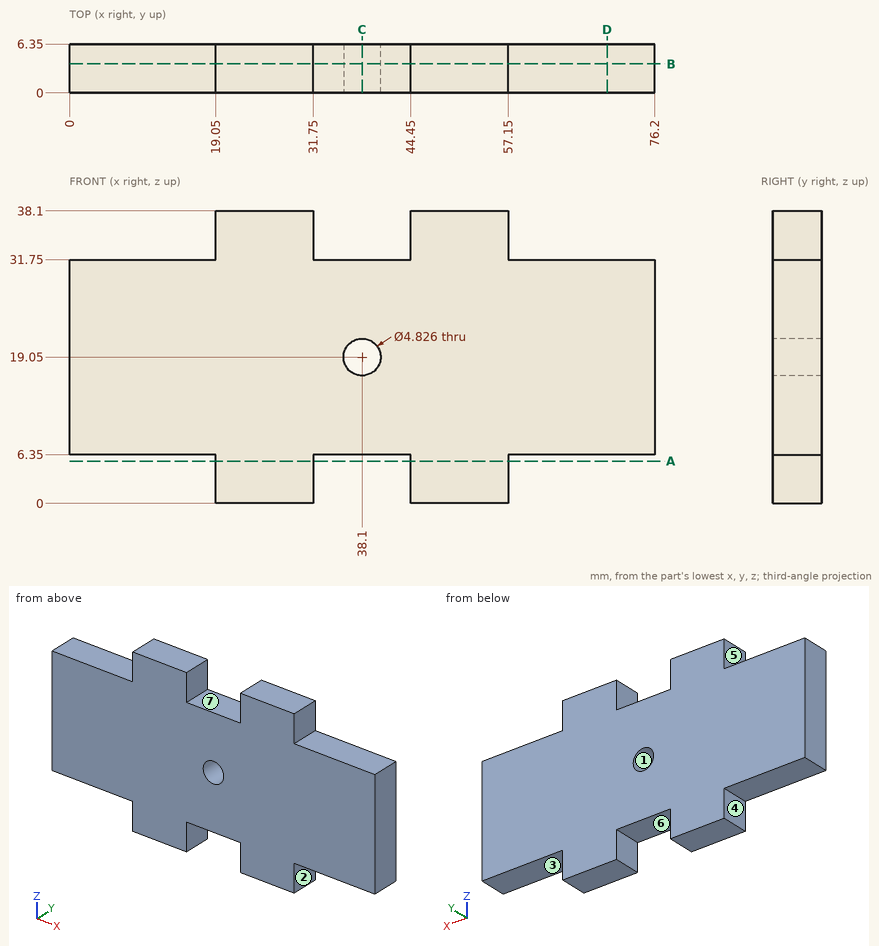
Geometry check sheet. Reference: drawing and pictorial views, mm from the part's lowest x, y, z. A direction names the side the tool comes from. Coordinates: 2 decimals unless noted, no trailing zeros. Write each loop counter-clockwise with the first axis right and the second up, starting at its lowest first coordinate (ties: lowest second). Pieces come first, ordered by that corner, then holes. Notation, with made-up numbers: (-23.75, 4.25) - (33.25, 4.25) arc R7 ccw to (33.25, 17.25) - close; hole circle Ø8 at (-7, 85.5). An arc over 180 degrees is marked (long way). One line per question, with ' | ' between items. Start each with the question number.
1. Draft check along X on the marked faces 1, 2 and 3. Enter one of: released by +X, released by -X, zero draft, split by the parting line, or undercut.
2. Material ranges on line 1 along Z through (x, y) = (38.1, 4); line 2 along X through (y, z) = (5, 4.5); line 3 along X through (y, z) = (4.75, 19.05), recorded low to high.
3. Access from +Z, -Z, +X, -X, +Y, -Y to the whole of each face (thin tool, end or side, straight path). Record for the marked faces 4, 5, 6 and 7.
4. Gauge pin test, flat ends, axial feed: P1, Ø3, axis at x = 70, y = 2, coming from the -Z side; P2, Ø4.5, axis at x = 38.1, z = 19.05, coming from the -Y side; P3, Ø1.9, axis at x = 69, y = 3.5, coming from the +Z side; P4, Ø3, axis at y = 4, z = 2.5, coming from the +X side. Record the tip position at first contact, or that the pin passes through.
5. Section check A-A (z = 5.5). Enter the section's corners in (x, y), plus the area to 3 significant figures.
6. Section check D-D (x = 70). Enter the section's corners in (y, z), plus the area to 3 significant figures.
7. Section check B-B (y = 3.75). Enter the section's corners in (x, z).
8. Section check C-C (x = 38.1). Enter the section's corners in (y, z), plus the area to 3 significant figures.
Computed values:
1) face 1: undercut | face 2: released by +X | face 3: zero draft
2) line 1: 6.35 to 16.64, 21.46 to 31.75 | line 2: 19.05 to 31.75, 44.45 to 57.15 | line 3: 0 to 35.69, 40.51 to 76.2
3) face 4: -Z, -X, +Y, -Y | face 5: +Z, -X, +Y, -Y | face 6: -Z, +Y, -Y | face 7: +Z, +Y, -Y
4) P1: z = 6.35 | P2: through | P3: z = 31.75 | P4: x = 57.15
5) outline: (19.05, 0) - (31.75, 0) - (31.75, 6.35) - (19.05, 6.35) - close; (44.45, 0) - (57.15, 0) - (57.15, 6.35) - (44.45, 6.35) - close | area: 161 mm²
6) outline: (0, 6.35) - (6.35, 6.35) - (6.35, 31.75) - (0, 31.75) - close | area: 161 mm²
7) outline: (0, 6.35) - (19.05, 6.35) - (19.05, 0) - (31.75, 0) - (31.75, 6.35) - (44.45, 6.35) - (44.45, 0) - (57.15, 0) - (57.15, 6.35) - (76.2, 6.35) - (76.2, 31.75) - (57.15, 31.75) - (57.15, 38.1) - (44.45, 38.1) - (44.45, 31.75) - (31.75, 31.75) - (31.75, 38.1) - (19.05, 38.1) - (19.05, 31.75) - (0, 31.75) - close; hole circle Ø4.83 at (38.1, 19.05)
8) outline: (0, 6.35) - (6.35, 6.35) - (6.35, 16.64) - (0, 16.64) - close; (0, 21.46) - (6.35, 21.46) - (6.35, 31.75) - (0, 31.75) - close | area: 131 mm²
